Source: CAD feature listing. Evaluate the final solid. Frame: model axes, mm. Face numbers are marked on the shaded views. A direction names the side the tool comes from. Round coordinates to 2 decimals unless told otherwise and drop trailing zeros. Loops run counter-clockwise (first coordinate to the right, second up) from the corner with the lowest first, then second, coordinate; pieces in that order, holes last. Notation, with made-up numbers: (66.25, 61) -> (78.25, 61) arc R24 ccw to (78.25, 77) -> close; hole circle Ø9 at (52, 86). An arc over 180 degrees is marked (long way). Write item = value, one per line.
from build123d import *

# Parameters (mm, degrees)
EXTRUDE_1_DEPTH      = 10
EXTRUDE_1_DEPTH_BACK = 10
SKETCH_1_R           = 25.4
EXTRUDE_2_DEPTH      = 1.5
SKETCH_3_W           = 54
SKETCH_3_H           = 44
EXTRUDE_3_DEPTH      = 3
SKETCH_4_R           = 3.1
CUT_EXTRUDE_1_DEPTH  = 3
FILLET_1_R           = 10
EXTRUDE_START        = 14
SKETCH_5_R           = 5
SKETCH_5_R_2         = 3.1
EXTRUDE_4_DEPTH      = 14


with BuildPart() as part:
    # 草图1 → 凸台-拉伸1 (new, two sides: drawn at the far end of the back side and taken through both)
    with BuildSketch(Plane.XY.offset(-EXTRUDE_1_DEPTH_BACK)):
        Circle(SKETCH_1_R)
    extrude(amount=EXTRUDE_1_DEPTH + EXTRUDE_1_DEPTH_BACK)

    # 草图2 → 凸台-拉伸2 (add)
    with BuildSketch(Plane.XY.offset(10)):
        with BuildLine():
            Line((-5, 0), (-5, 41.6))
            Line((-5, 41.6), (35, 41.6))
            Line((35, 41.6), (5, 0))
            ThreePointArc((5, 0), (0, -5), (-5, 0))
        make_face()
    extrude_2 = extrude(amount=EXTRUDE_2_DEPTH)

    # 镜向1: 凸台-拉伸2 across plane
    add(extrude_2.mirror(Plane.XY))

    # 草图3 → 凸台-拉伸3 (add)
    with BuildSketch(Plane(origin=(0, 41.6, 0), x_dir=(1, 0, 0), z_dir=(0, 1, 0))):
        with Locations((19, 0)):
            Rectangle(SKETCH_3_W, SKETCH_3_H)
    extrude(amount=EXTRUDE_3_DEPTH)

    # 草图4 → 切除-拉伸1 (cut)
    with BuildSketch(Plane(origin=(0, 44.6, 0), x_dir=(1, 0, 0), z_dir=(0, 1, 0))):
        with Locations(Location((-1, 15, 0), (0, 0, 270))):
            Circle(SKETCH_4_R)
        with Locations(Location((39, 15, 0), (0, 0, 270))):
            Circle(SKETCH_4_R)
        with Locations(Location((39, -15, 0), (0, 0, 270))):
            Circle(SKETCH_4_R)
        with Locations(Location((-1, -15, 0), (0, 0, 270))):
            Circle(SKETCH_4_R)
    extrude(amount=-CUT_EXTRUDE_1_DEPTH, mode=Mode.SUBTRACT)

    # 圆角1
    fillet_1_edges = [part.edges().sort_by_distance(p)[0] for p in [
        (-8, 43.1, -22),
        (-8, 43.1, 22),
        (46, 43.1, 22),
        (46, 43.1, -22),
    ]]
    fillet(fillet_1_edges, radius=FILLET_1_R)

    # 草图5 → 凸台-拉伸4 (add)
    # profile 1 of 4: a face of its own
    with BuildSketch(Plane(origin=(0, 44.6, 0), x_dir=(1, 0, 0), z_dir=(0, 1, 0)).offset(EXTRUDE_START)):
        with Locations(Location((-1, 15, 0), (0, 0, 270))):
            Circle(SKETCH_5_R)
        with Locations(Location((-1, 15, 0), (0, 0, 270))):
            Circle(SKETCH_5_R_2, mode=Mode.SUBTRACT)
    # profile 2 of 4: a face of its own
    with BuildSketch(Plane(origin=(0, 44.6, 0), x_dir=(1, 0, 0), z_dir=(0, 1, 0)).offset(EXTRUDE_START)):
        with Locations(Location((39, 15, 0), (0, 0, 270))):
            Circle(SKETCH_5_R)
        with Locations(Location((39, 15, 0), (0, 0, 270))):
            Circle(SKETCH_5_R_2, mode=Mode.SUBTRACT)
    # profile 3 of 4: a face of its own
    with BuildSketch(Plane(origin=(0, 44.6, 0), x_dir=(1, 0, 0), z_dir=(0, 1, 0)).offset(EXTRUDE_START)):
        with Locations(Location((-1, -15, 0), (0, 0, 270))):
            Circle(SKETCH_5_R)
        with Locations(Location((-1, -15, 0), (0, 0, 270))):
            Circle(SKETCH_5_R_2, mode=Mode.SUBTRACT)
    # profile 4 of 4: a face of its own
    with BuildSketch(Plane(origin=(0, 44.6, 0), x_dir=(1, 0, 0), z_dir=(0, 1, 0)).offset(EXTRUDE_START)):
        with Locations(Location((39, -15, 0), (0, 0, 270))):
            Circle(SKETCH_5_R)
        with Locations(Location((39, -15, 0), (0, 0, 270))):
            Circle(SKETCH_5_R_2, mode=Mode.SUBTRACT)
    extrude(amount=-EXTRUDE_4_DEPTH)


solid = part.part
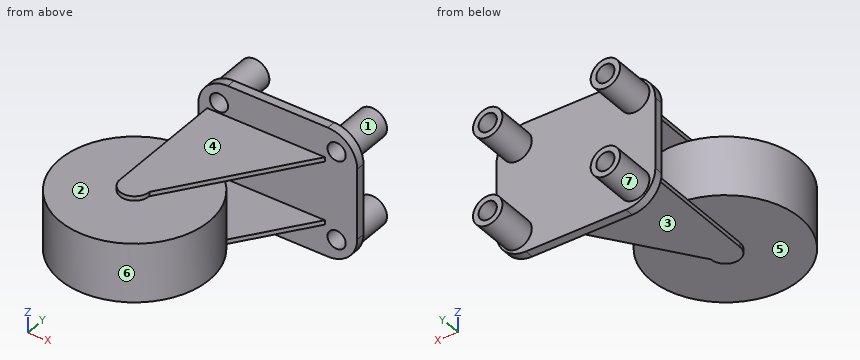
1. Contact query for flat-ended pins moving along their axis: pin 1 Ø1 at (x, y) = (24.5, 7.5) entering from -Z; pin 2 Ø5 at (y, z) = (45, 7.5) entering from -X; pin 3 Ø22 at (x, z) = (23.5, -10.5) entering from +Y; pin 4 Ø3.5 at (x, z) = (39, -15) entering from -Y. Output: stop coordinate, or through.
Evaluation:
pin_1 = -10
pin_2 = -8
pin_3 = 44.6
pin_4 = through
2. Set-up query: the marked faces 1, 2, 3 and 4. Return all of +Z, -Z, +X, -X, +Y, -Y with unobstructed straight access to the full face (end or side cutting, diameter ignored); none if empty.
Evaluation:
face_1 = +Y
face_2 = +Z, -Y
face_3 = -Z, +X, -X, -Y
face_4 = +Z, +X, -X, -Y
3. Mould query, pull axis X, two halves, no side actions, for the marked faces 5, 6 and 7. Classes: released by +X, released by -X, zero draft, split by the parting line, or undercut.
Evaluation:
face_5 = zero draft
face_6 = split by the parting line
face_7 = undercut
4. Section query C-C (z = -15). Return the cut outline in (x, y), then the cut area to 3 significant figures.
Evaluation:
outline = (-7.54, 41.6) -> (-4.1, 41.6) -> (-4.1, 58.6) -> (-6, 58.6) -> (-6, 44.6) -> (-7.54, 44.6) -> close; (2.1, 41.6) -> (35.9, 41.6) -> (35.9, 58.6) -> (34, 58.6) -> (34, 44.6) -> (4, 44.6) -> (4, 58.6) -> (2.1, 58.6) -> close; (42.1, 41.6) -> (45.54, 41.6) -> (45.54, 44.6) -> (44, 44.6) -> (44, 58.6) -> (42.1, 58.6) -> close
area = 228 mm²
5. Section query D-D (x = -1). Give the number of separate pieces and of enclosed holes in the cut face, then the cut area to 3 significant figures.
Evaluation:
separate_pieces = 3
enclosed_holes = 1
area = 1,350 mm²
6. Section query A-A (z = -4). Return the cut outline in (x, y), then the cut area to 3 significant figures.
Evaluation:
outline = circle Ø50.8 at (0, 0); (-8, 41.6) -> (46, 41.6) -> (46, 44.6) -> (-8, 44.6) -> close
area = 2,190 mm²
7. Line query: probe 1 along X at (y, z) = (52.5, 15); probe 2 along Y at (x, z) = (1, 9.5); probe 3 along Y at (x, z) = (29, -19.5). Output: solid intervals per line, ascending. Write a range as from..to.
Evaluation:
probe_1 = -6..-4.1, 2.1..4, 34..35.9, 42.1..44
probe_2 = -25.38..25.38, 41.6..44.6
probe_3 = 41.6..44.6
8. Section query B-B (x = 39). Return the cut outline in (y, z).
Evaluation:
outline = (41.6, -21.54) -> (44.6, -21.54) -> (44.6, -20) -> (58.6, -20) -> (58.6, -18.1) -> (41.6, -18.1) -> close; (41.6, -11.9) -> (58.6, -11.9) -> (58.6, -10) -> (44.6, -10) -> (44.6, 10) -> (58.6, 10) -> (58.6, 11.9) -> (41.6, 11.9) -> close; (41.6, 18.1) -> (58.6, 18.1) -> (58.6, 20) -> (44.6, 20) -> (44.6, 21.54) -> (41.6, 21.54) -> close
